Autodesk Fusion 360 part; units mm, degrees
sketch "Sketch1" plane through (0, 0, 0) normal (0, 0, 1) x (1, 0, 0)
  circle A0 centre (0, 0) radius 4.65
  circle A1 centre (0, 0) radius 10
  line L0 (-33.85, -25.2927) -> (33.85, -25.2927)
  circle A2 centre (33.85, -25.2927) radius 5.7
  circle A3 centre (-33.85, -25.2927) radius 5.7
  line L1 (-33.85, -30.9927) -> (33.85, -30.9927)
  line L2 (-33.85, -19.5927) -> (33.85, -19.5927)
  line L3 (10, -19.5927) -> (10, 0)
  line L4 (-10, -19.5927) -> (-10, 0)
  line L5 (0.7275, -4.5927) -> (0.7275, -19.5927) construction
  line L6 (0, 0) -> (0, -19.5927) construction
  dimension "d2" = 9.3
  dimension "d3" = 20
  dimension "d9" = 67.7
  dimension "d13" = 11.4
  dimension "d14" = 11.4
  dimension "d37" = 15
extrude "Extrude1" add sketch "Sketch1" along normal blind 5 contours A1 makes body 1
extrude "Extrude2" add sketch "Sketch1" along normal blind 5 contours A1 L2 L3 L4 bodies 1
extrude "Extrude3" add sketch "Sketch1" against normal blind 40 separate body contours L0 A2 A3 L2 | A2 | A3 | L0 A2 A3 L1 makes body 2
extrude "Extrude4" add 1 faces at (-3.3333, -19.5927, 1.6667) along direction (0, -1, 0) blind 0.2 on bodies 1 bodies 1 2
chamfer "Chamfer1" distance 5 distance2 10.8 1 edges at (0, -19.7927, 0) measured on face at (-3.3333, -19.7927, 1.6667) on bodies 1
hole "Hole1" at (-33.85, -25.2927, 0) at (33.85, -25.2927, 0) direction (0, 0, -1) diameter 5.4 depth 38 tip angle 180 bodies 1
hole "Hole2" at (33.85, -25.2927, -38) direction (0, 0, -1) diameter 2.65 depth 2 tip angle 180 countersink diameter 5 countersink angle 90 bodies 1
hole "Hole3" at (-33.85, -25.2927, -38) direction (0, 0, -1) diameter 2.65 depth 2 tip angle 180 countersink diameter 5 countersink angle 90 bodies 1
sketch "Sketch2" plane through (0, -30.9927, 0) normal (0, -1, 0) x (1, 0, 0)
  line L0 (33.85, 0) -> (-33.85, 0)
  line L1 (-33.85, 0) -> (-33.85, -40)
  line L2 (-33.85, -40) -> (33.85, -40)
  line L3 (33.85, -40) -> (33.85, 0)
  line L4 (-33.85, -40) -> (-28.15, -40) construction
  line L5 (33.85, -40) -> (28.15, -40) construction
  arc A0 (28.15, -40) -> (-28.15, -40) centre (0, -38.1329) ccw
  dimension "d39" = 5.7
  dimension "d40" = 5.7
extrude "Extrude5" cut sketch "Sketch2" against normal up to surface (11.4 mm away) contours L2 A0 bodies 1
equation "stemdia = 9.2 mm"
equation "d2 = stemdia + 0.1 mm"
equation "screwwidth = 67.7 mm"
equation "screwheight = 5.6 mm"
equation "d9 = screwwidth"
equation "shiftscrewdia = 2.55 mm"
equation "shiftiscrewdepth = 2 mm"
equation "d13 = standoffwidth"
equation "d14 = standoffwidth"
equation "standoff = 40 mm"
equation "d23 = standoff - 2 mm"
equation "d36 = ( 5.5 * 2 ) * 1 mm - 0.2 mm"
equation "standoffwidth = 11.4 mm"
equation "d39 = standoffwidth / 2"
equation "d40 = standoffwidth / 2"
For this review, take the finished solid that the model builds, in its own axes (mm). A direction names the side the tool comes from. Coordinates: 2 decimals unless noted, no trailing zeros. Write each loop counter-clockwise with the first axis right and the second up, starting at its lowest first coordinate (ties: lowest second). Pieces come first, ordered by that corner, then holes.
(1) Add section D-D on z = -30. Give the boundary of the cut face in (x, y).
(2) For pin 1 Ø2.5 at (y, z) = (-20, 3) entering from -X; pin 2 Ø1.5 at (x, y) = (9, -24) entering from -Z; pin 3 Ø10 at (x, y) = (-4.5, -5) entering from -Z; pin 4 Ø6 at (x, y) = (31.5, -18.5) entering from -Z, all flat-tipped, find the tip position at first contact; note any pin that passes through.
(3) Wall thickness on probe 1 along Y at (x, z) = (-33.85, -23); probe 2 along Z at (x, y) = (1, 5.5); probe 3 along Z at (x, y) = (29, -22.5): over which ranges is each line inside the solid? List them lowest first.
(4) The part is to be moulded in two halves that separate along Y. For faces 4 (the face through (39.55, -25.42, -19.72)), 5 (the face through (0, -19.593, -6)), 6 (the face through (33.79, -23.97, -39.59)), say which applies: +Y half, -Y half, draft (parallel to the pull), parting line (faces both ways), or undercut.
(5) Add section A-A on z = -15. Give the boundary of the cut face in (x, y).
(6) Tool access review of faces 1 (the face through (31.173, -24.941, -19.266)), 2 (the face through (10, -12, 2)), 3 (the face through (-10, -12, 2)): name each direction out of +Z, -Z, +X, -X, +Y, -Y from which nothing blocks a thin tool from reaching the whole face with its end or side.
(7) Add section C-C on z = -5.5. Give the boundary of the cut face in (x, y), then the cut area to 3 significant figures.
Answer sheet:
1. outline: (-33.85, -30.99) - (-27.01, -30.99) - (-27.01, -19.59) - (-33.85, -19.59) arc R5.7 ccw to start; (27.01, -30.99) - (33.85, -30.99) arc R5.7 ccw to (33.85, -19.59) - (27.01, -19.59) - close; hole circle Ø5.4 at (-33.85, -25.29); hole circle Ø5.4 at (33.85, -25.29)
2. pin 1: stops at x = -10
2. pin 2: stops at z = -11.66
2. pin 3: stops at z = 0
2. pin 4: stops at z = -40
3. probe 1: y = -30.99 to -27.99, -22.59 to -19.59
3. probe 2: z = 0 to 5
3. probe 3: z = -40 to 0
4. face 4: parting line
4. face 5: +Y half
4. face 6: undercut
5. outline: (-33.85, -30.99) - (-16.15, -30.99) - (-16.15, -19.59) - (-33.85, -19.59) arc R5.7 ccw to start; (16.15, -30.99) - (33.85, -30.99) arc R5.7 ccw to (33.85, -19.59) - (16.15, -19.59) - close; hole circle Ø5.4 at (-33.85, -25.29); hole circle Ø5.4 at (33.85, -25.29)
6. face 1: +Z
6. face 2: +Z, +X, +Y, -Y
6. face 3: +Z, -X, +Y, -Y
7. outline: (-33.85, -30.99) - (33.85, -30.99) arc R5.7 ccw to (33.85, -19.59) - (-33.85, -19.59) arc R5.7 ccw to start; hole circle Ø5.4 at (-33.85, -25.29); hole circle Ø5.4 at (33.85, -25.29)
7. area: 828 mm2
